```python
from build123d import *

# Parameters (mm, degrees)
EXTRUDE_4_DEPTH      = 5.5
SKETCH_8_R           = 2.925
CUT_EXTRUDE_8_DEPTH  = 4.05
SKETCH_9_R           = 1
CUT_EXTRUDE_9_DEPTH  = 17.451421165
SKETCH_10_R          = 1
CUT_EXTRUDE_10_DEPTH = 17.025035362


with BuildPart() as part:
    # 草图1 → 凸台-拉伸4 (new body)
    with BuildSketch(Plane(origin=(0, 0, 0), x_dir=(1, 0, 0), z_dir=(0, 1, 0))):
        with BuildLine():
            ThreePointArc((3.662209834, 0), (2.331674388, 2.824017602), (-0.693125212, 3.596019787))
            Line((-0.693125212, 3.596019787), (-0.693125212, 0))
            Line((-0.693125212, 0), (3.662209834, 0))
        make_face()
        with BuildLine():
            Line((-0.693125212, 0), (-0.693125212, 3.596019787))
            ThreePointArc((-0.693125212, 3.596019787), (-2.824017602, 2.331674388), (-3.662209834, 0))
            Line((-3.662209834, 0), (-0.693125212, 0))
        make_face()
        with BuildLine():
            Line((3.662209834, 0), (-0.693125212, 0))
            Line((-0.693125212, 0), (-0.693125212, -3.596019787))
            ThreePointArc((-0.693125212, -3.596019787), (2.331674388, -2.824017602), (3.662209834, 0))
        make_face()
        with BuildLine():
            Line((-0.693125212, -3.596019787), (-0.693125212, 0))
            Line((-0.693125212, 0), (-3.662209834, 0))
            ThreePointArc((-3.662209834, 0), (-2.824017602, -2.331674388), (-0.693125212, -3.596019787))
        make_face()
        with BuildLine():
            ThreePointArc((-3.662209834, 0), (-2.824017602, 2.331674388), (-0.693125212, 3.596019787))
            Line((-0.693125212, 3.596019787), (-14.255367792, 0.9819262))
            ThreePointArc((-14.255367792, 0.9819262), (-15.066103593, 0), (-14.255367792, -0.9819262))
            Line((-14.255367792, -0.9819262), (-0.693125212, -3.596019787))
            ThreePointArc((-0.693125212, -3.596019787), (-2.824017602, -2.331674388), (-3.662209834, 0))
        make_face()
    extrude(amount=EXTRUDE_4_DEPTH)

    # 草图8 → 切除-拉伸8 (cut)
    with BuildSketch(Plane(origin=(0, 5.5, 0), x_dir=(1, 0, 0), z_dir=(0, 1, 0))):
        with Locations(Location((0, 0, 0), (0, 0, 270))):
            Circle(SKETCH_8_R)
    extrude(amount=-CUT_EXTRUDE_8_DEPTH, mode=Mode.SUBTRACT)

    # 草图9 → 切除-拉伸9 (cut, through all)
    with BuildSketch(Plane(origin=(0, 5.5, 0), x_dir=(1, 0, 0), z_dir=(0, 1, 0))):
        with Locations(Location((-10.814314949, 0, 0), (0, 0, 270))):
            Circle(SKETCH_9_R)
    extrude(amount=-CUT_EXTRUDE_9_DEPTH, mode=Mode.SUBTRACT)

    # 草图10 → 切除-拉伸10 (cut, through all)
    with BuildSketch(Plane(origin=(0, 1.45, 0), x_dir=(1, 0, 0), z_dir=(0, 1, 0))):
        with Locations(Location((0, 0, 0), (0, 0, 270))):
            Circle(SKETCH_10_R)
    extrude(amount=-CUT_EXTRUDE_10_DEPTH, mode=Mode.SUBTRACT)


solid = part.part
```
Here's how the part is built. I have some questions about the finished solid (model axes, mm). A direction names the side the tool comes from. Round coordinates to 2 decimals unless told otherwise and drop trailing zeros. Write each loop counter-clockwise with the first axis right and the second up, starting at its lowest first coordinate (ties: lowest second). Pieces come first, ordered by that corner, then holes.
Q1. If we mould it in two halves opening along X, with no side actions, what happens to faces 1 (the cylindrical face through (-2.595, 3.503, 1.35)), 2 (the flat face through (-4, 0, 0)), 3 (the flat face through (-7.379, 2.712, -2.307))? For each: +X half, -X half, draft (parallel to the pull), parting line (faces both ways), or undercut.
Q2. Please list where these lines run through material, in increasing order: probe 1 along X at (y, z) = (4.1, 0) (3 decimals); probe 2 along X at (y, z) = (0.4, 0); probe 3 along Y at (x, z) = (-0.5, -1.25).
Q3. If we section it at C-C on z = -2.75: Write out the boundary of the cut face in (x, y).
Q4. Which directions (+Z, -Z, +X, -X, +Y, -Y) give clear straight access to the entire face, cutting with the end or side of a thin tool? Please do faces 4 (the flat face through (-1.3, 1.45, 0)), 5 (the cylindrical face through (-11.79, 2.79, -0.22)).
Q5. If we section it at D-D on x = -11.25: Write out the boundary of the cut face in (y, z), plus the area to 3 significant figures.
Q6. If we section it at A-A on x = 0: Write out the boundary of the cut face in (y, z) (3 decimals).
Q7. If we section it at B-B on y = 4.6: Write out the boundary of the cut face in (x, z) (3 decimals).
Q8. Will this pin go through, and if not, where does the flat tip stop? P1, Ø1.8, axis at x = 0, z = 0, coming from the +Y side.
Answer below:
1. face 1: undercut
1. face 2: draft
1. face 3: -X half
2. probe 1: x = -15.066 to -11.814, -9.814 to -2.925, 2.925 to 3.662
2. probe 2: x = -15.07 to -11.81, -9.81 to -1, 1 to 3.66
2. probe 3: y = 0 to 1.45
3. outline: (-5.08, 0) - (2.42, 0) - (2.42, 5.5) - (1, 5.5) - (1, 1.45) - (-1, 1.45) - (-1, 5.5) - (-5.08, 5.5) - close
4. face 4: +Y
4. face 5: +Y, -Y
5. outline: (0, -1.56) - (5.5, -1.56) - (5.5, -0.9) - (0, -0.9) - close; (0, 0.9) - (5.5, 0.9) - (5.5, 1.56) - (0, 1.56) - close
5. area: 7.27 mm2
6. outline: (0, -3.662) - (5.5, -3.662) - (5.5, -2.925) - (1.45, -2.925) - (1.45, -1) - (0, -1) - close; (0, 1) - (1.45, 1) - (1.45, 2.925) - (5.5, 2.925) - (5.5, 3.662) - (0, 3.662) - close
7. outline: (-14.255, -0.982) - (-0.693, -3.596) arc R3.662 ccw (long way) to (-0.693, 3.596) - (-14.255, 0.982) arc R1 ccw to start; hole circle Ø2 at (-10.814, 0); hole circle Ø5.85 at (0, 0)
8. P1: passes through
